```python
from build123d import *

# Parameters (mm, degrees)
SKETCH1_W               = 60
SKETCH1_H               = 60
BOSS_EXTRUDE1_DEPTH     = 60
SKETCH1_3_R             = 30
BOSS_EXTRUDE2_DEPTH     = 120
CUT_EXTRUDE1_START      = 120
SKETCH1_4_W             = 20
SKETCH1_4_H             = 20
CUT_EXTRUDE1_DEPTH      = 20
SKETCH1_5_R             = 10
CUT_EXTRUDE2_DEPTH      = 128.279220614
CUT_EXTRUDE3_DEPTH      = 138.477270849
CUT_EXTRUDE3_DEPTH_BACK = 138.477270849


with BuildPart() as part:
    # Sketch1 → Boss-Extrude1 (new body)
    with BuildSketch(Plane(origin=(0, 0, 0), x_dir=(1, 0, 0), z_dir=(0, 1, 0))):
        Rectangle(SKETCH1_W, SKETCH1_H)
    extrude(amount=BOSS_EXTRUDE1_DEPTH)

    # Sketch1<3> → Boss-Extrude2 (add)
    with BuildSketch(Plane(origin=(0, 0, 0), x_dir=(1, 0, 0), z_dir=(0, 1, 0))):
        with Locations(Location((0, 0, 0), (0, 0, 270))):
            Circle(SKETCH1_3_R)
    extrude(amount=BOSS_EXTRUDE2_DEPTH)

    # Sketch1<4> → Cut-Extrude1 (cut)
    with BuildSketch(Plane(origin=(0, 0, 0), x_dir=(1, 0, 0), z_dir=(0, 1, 0)).offset(CUT_EXTRUDE1_START)):
        Rectangle(SKETCH1_4_W, SKETCH1_4_H)
    extrude(amount=-CUT_EXTRUDE1_DEPTH, mode=Mode.SUBTRACT)

    # Sketch1<5> → Cut-Extrude2 (cut, through all)
    with BuildSketch(Plane(origin=(0, 0, 0), x_dir=(1, 0, 0), z_dir=(0, 1, 0))):
        with Locations(Location((0, 0, 0), (0, 0, 270))):
            Circle(SKETCH1_5_R)
    extrude(amount=CUT_EXTRUDE2_DEPTH, mode=Mode.SUBTRACT)

    # Sketch2 → Cut-Extrude3 (cut, two sides: drawn at the far end of the back side and taken through both)
    with BuildSketch(Plane.XY.offset(30).offset(-CUT_EXTRUDE3_DEPTH_BACK)):
        Polygon((-110.366799799, -100.733599598), (-30, 60), (0, 120), (30, 60), (110.366799799, -100.733599598), (110.366799799, 258.677655371), (-110.366799799, 258.677655371), align=None)
    extrude(amount=CUT_EXTRUDE3_DEPTH + CUT_EXTRUDE3_DEPTH_BACK, mode=Mode.SUBTRACT)


solid = part.part
```
CAD build for the part. Positions are in the model's coordinates, mm. A direction names the side the tool comes from. Coordinates: 2 decimals unless noted, no trailing zeros. Order: outer loops, then holes, each group sorted by start corner. A loop starts at its lowest first (then second) coordinate and runs counter-clockwise, first axis right, second up. Notation, with made-up numbers: (72.25, -20.75) -> (105.25, -20.75) arc R26 cw to (105.25, 3.25) -> close; hole circle Ø5 at (1.5, 64). An arc over 180 degrees is marked (long way). Use one line per item in the form item = value. Start each with the question number.
1) Band-saw the part on C-C on z = 25. Give the cut face in (x, y).
2) Band-saw the part on A-A on y = 24. Give the cut face in (x, z), then the cut area to 3 significant figures.
3) Band-saw the part on D-D on x = 25.5. Give the cut face in (y, z), then the cut area to 3 significant figures.
4) Band-saw the part on B-B on x = 5. Give the cut face in (y, z).
5) Drop flat-ended pins along their axis: pin 1 (12 mm diameter, centred on x = 19, z = -3, fed in from -Y); pin 2 (3 mm diameter, centred on x = -3.5, z = 7, fed in from +Y); pin 3 (3 mm diameter, centred on x = 6.5, z = 7, fed in from +Y); pin 4 (6 mm diameter, centred on x = 4.5, y = 115, fed in from +Z). Give the stop position or say it passes through.
6) Drill centre lines: L1, parallel to X at y = 54.5, z = 0; L2, parallel to Y at x = -9.5, z = -7. Where is each one in solid material? Low to high. Write a range as [from, to].
7) Pull direction Z, two halves, no side cores. Call faces 4 (the flat face through (15, 90, 0)), 5 (the flat face through (-8, 100, 8)), 6 (the flat face through (0, 30, 30)), 7 (the flat face through (0, 30, -30)): +Z half, -Z half, draft (parallel to the pull), parting line (faces both ways), or undercut.
8) Tool access for faces 1 (the flat face through (8, 100, 8)), 2 (the cylindrical face through (0, 77, 30)), 3 (the flat face through (-24, 60, 23)): list every direction of +Z, -Z, +X, -X, +Y, -Y with a clear straight run to the whole face (end or side of a thin tool).
Entries:
q1.outline = (-30, 0) -> (30, 0) -> (30, 60) -> (16.58, 60) -> (16.58, 86.83) -> (0, 120) -> (-16.58, 86.83) -> (-16.58, 60) -> (-30, 60) -> close
q2.outline = (-30, -30) -> (30, -30) -> (30, 30) -> (-30, 30) -> close; hole circle Ø20 at (0, 0)
q2.area = 3,290 mm2
q3.outline = (0, -30) -> (60, -30) -> (60, -15.8) -> (69, -15.8) -> (69, 15.8) -> (60, 15.8) -> (60, 30) -> (0, 30) -> close
q3.area = 3,880 mm2
q4.outline = (0, -30) -> (60, -30) -> (60, -29.58) -> (110, -29.58) -> (110, -10) -> (100, -10) -> (100, -8.66) -> (0, -8.66) -> close; (0, 8.66) -> (100, 8.66) -> (100, 10) -> (110, 10) -> (110, 29.58) -> (60, 29.58) -> (60, 30) -> (0, 30) -> close
q5.pin_1 = 0
q5.pin_2 = through
q5.pin_3 = 100
q5.pin_4 = 29.96
q6.L1 = [-30, -10], [10, 30]
q6.L2 = [0, 100]
q7.face_4 = draft
q7.face_5 = undercut
q7.face_6 = +Z half
q7.face_7 = -Z half
q8.face_1 = +X, -X, +Y
q8.face_2 = +Z, +Y
q8.face_3 = +Z, -X, +Y
